Work out the finished part from the listing and answer in its coordinate system (mm). A direction names the side the tool comes from. Coordinates: 2 decimals unless noted, no trailing zeros. Loops run counter-clockwise (first coordinate to the right, second up) from the corner with the lowest first, then second, coordinate; pieces in that order, holes last. Notation, with made-up numbers: (-10, 12.5) - (39, 12.5) arc R16 ccw to (39, 42.5) - close; hole circle Ø9 at (-18.5, 42). An arc over 180 degrees is marked (long way). Write each question's results on one line, items separated by ' | '. Start each with the question number.
1. A cutting plane is placed at C-C on y = 54. Determine the outline of the cut face in (x, z).
2. Determine the mould class of faces 3 (the flat face through (-478.912, 49, -10)), 4 (the flat face through (478.912, 49, 10)), 5 (the flat face through (6, 49, -674)), 6 (the flat face through (-7, 49, 694)) for opening direction X: released by +X, released by -X, zero draft, split by the parting line, or undercut.
3. This flat-tipped pin is pushed along its axis until it touches: P1, Ø9, axis at y = 75, z = 654, coming from the +X side. Where does it stop, or does it pass through?
4. A cutting plane is placed at A-A on x = 191. Determine the outline of the cut face in (y, z), then the cut area to 3 significant figures.
5. A cutting plane is placed at B-B on z = -423. Determine the outline of the cut face in (x, y).
6. Which of the six approach directions +Z, -Z, +X, -X, +Y, -Y give full straight-line access (tool end or side, diameter ignored) to faces 1 (the flat face through (463, 0, 3)), 2 (the flat face through (-458.912, 49, -9))?
7. Find the intervals of material crossed by line 1 along Y through (x, z) = (-472.5, 654); line 2 along Z through (x, y) = (-471, 75); line 3 along X through (y, z) = (25, -686), in increasing order. Write a range as [from, to].
Autodesk Inventor part; units mm, degrees
ref_plane "YZ Plane" through (0, 0, 0) normal (1, 0, 0) x (0, 1, 0)
ref_plane "XZ Plane" through (0, 0, 0) normal (0, 1, 0) x (-1, 0, 0)
ref_plane "XY Plane" through (0, 0, 0) normal (0, 0, 1) x (1, 0, 0)
sketch "Sketch1" plane through (0, 0, 0) normal (0, 1, 0) x (-1, 0, 0)
  line L0 (478.912, 694) -> (-478.912, 694)
  line L1 (-478.912, 694) -> (-478.912, -694)
  line L2 (-478.912, -694) -> (478.912, -694)
  line L3 (478.912, -694) -> (478.912, 694)
  line L4 (478.912, 694) -> (-478.912, -694) construction
  line L5 (-478.912, 694) -> (478.912, -694) construction
  line L6 (458.912, 674) -> (-458.912, 674)
  line L7 (-458.912, 674) -> (-458.912, -674)
  line L8 (-458.912, -674) -> (458.912, -674)
  line L9 (458.912, -674) -> (458.912, 674)
  line L10 (458.912, 674) -> (-458.912, -674) construction
  line L11 (-458.912, 674) -> (458.912, -674) construction
  point P0 (0, 0)
  point P1 (458.912, 0)
  point P2 (-448.912, 0)
  point P3 (-458.912, 0)
  point P4 (0, 674)
  point P5 (0, -674)
  dimension "d0" = 957.824
  dimension "d1" = 1388
  dimension "d2" = 917.824
  dimension "d3" = 1348
extrude "Extrusion7" add sketch "Sketch1" along normal blind 100
sketch "Sketch2" plane through (478.912, 0, 694) normal (1, 0, 0) x (0, 0, -1)
  line L0 (0, 0) -> (0, 100)
  line L1 (0, 100) -> (1388, 100)
  point P0 (694, 0)
  point P1 (40, 75)
  dimension "d40" = 40
  dimension "d41" = 25
hole "Hole1" at (478.912, 75, 654) direction (-1, 0, 0) diameter 8 end through all
sketch "Sketch3" plane through (478.912, 0, 694) normal (1, 0, 0) x (0, 0, -1)
  line L0 (0, 0) -> (0, 100)
  line L1 (0, 0) -> (1388, 0)
  point P0 (694, 0)
  point P1 (40, 25)
  dimension "d42" = 40
  dimension "d43" = 25
hole "Hole2" at (478.912, 25, 654) direction (-1, 0, 0) diameter 8 end through all
sketch "Sketch4" plane through (478.912, 0, 694) normal (1, 0, 0) x (0, 0, -1)
  line L0 (1388, 0) -> (1388, 100)
  line L1 (0, 100) -> (1388, 100)
  point P0 (694, 0)
  point P1 (1348, 75)
  dimension "d58" = 40
  dimension "d59" = 25
hole "Hole3" at (478.912, 75, -654) direction (-1, 0, 0) diameter 8 end through all
sketch "Sketch5" plane through (478.912, 0, 694) normal (1, 0, 0) x (0, 0, -1)
  line L0 (1388, 0) -> (1388, 100)
  line L1 (0, 0) -> (1388, 0)
  point P0 (694, 0)
  point P1 (1348, 25)
  dimension "d60" = 40
  dimension "d61" = 25
hole "Hole4" at (478.912, 25, -654) direction (-1, 0, 0) diameter 8 end through all
sketch "Sketch6" plane through (-478.912, 0, 694) normal (0, 0, 1) x (1, 0, 0)
  line L0 (0, 100) -> (957.824, 100)
  line L1 (957.824, 0) -> (957.824, 100)
  line L2 (0, 0) -> (957.824, 0)
  point P0 (478.912, 0)
  point P1 (917.824, 75)
  point P2 (917.824, 25)
  dimension "d69" = 25
  dimension "d70" = 40
  dimension "d71" = 40
  dimension "d72" = 25
hole "Hole5" at (438.912, 75, 694) at (438.912, 25, 694) direction (0, 0, -1) diameter 8 end through all
sketch "Sketch7" plane through (-478.912, 0, 694) normal (0, 0, 1) x (1, 0, 0)
  line L0 (0, 0) -> (0, 100)
  line L1 (0, 100) -> (957.824, 100)
  point P0 (478.912, 0)
  point P1 (40, 75)
  dimension "d87" = 40
  dimension "d88" = 25
hole "Hole6" at (-438.912, 75, 694) direction (0, 0, -1) diameter 8 end through all
sketch "Sketch8" plane through (-478.912, 0, 694) normal (0, 0, 1) x (1, 0, 0)
  line L0 (0, 0) -> (0, 100)
  line L1 (0, 0) -> (957.824, 0)
  point P0 (478.912, 0)
  point P1 (40, 25)
  dimension "d89" = 40
  dimension "d90" = 25
hole "Hole7" at (-438.912, 25, 694) direction (0, 0, -1) diameter 8 end through all
properties part number "solar panels holder 2"
Values:
1) outline: (-478.91, -694) - (478.91, -694) - (478.91, 694) - (-478.91, 694) - close; hole (-458.91, -674) - (458.91, -674) - (458.91, 674) - (-458.91, 674) - close
2) face 3: released by -X | face 4: released by +X | face 5: undercut | face 6: zero draft
3) P1: x = 478.91
4) outline: (0, -694) - (100, -694) - (100, -674) - (0, -674) - close; (0, 674) - (100, 674) - (100, 694) - (0, 694) - close | area: 4,000 mm^2
5) outline: (-478.91, 0) - (-458.91, 0) - (-458.91, 100) - (-478.91, 100) - close; (458.91, 0) - (478.91, 0) - (478.91, 100) - (458.91, 100) - close
6) face 1: +Z, -Z, +X, -X, -Y | face 2: +Y, -Y
7) line 1: [0, 21], [29, 71], [79, 100] | line 2: [-694, -658], [-650, 650], [658, 694] | line 3: [-478.91, -442.91], [-434.91, 434.91], [442.91, 478.91]
